Source: CAD feature listing. Evaluate the final solid. Frame: model axes, mm. Coordinates: 2 decimals unless noted, no trailing zeros. Order: outer loops, then holes, each group sorted by start corner. A loop starts at its lowest first (then second) coordinate and runs counter-clockwise, first axis right, second up.
```python
from build123d import *

# Parameters (mm, degrees)
SKETCH1_R               = 6
SKETCH1_R_2             = 15
BOSS_EXTRUDE1_DEPTH     = 5
FILLET1_R               = 5
SKETCH3_R               = 2.1
CUT_EXTRUDE1_DEPTH      = 352.212186577
CIRPATTERN1_COUNT       = 4
CUT_EXTRUDE2_DEPTH      = 352.212186577
CUT_EXTRUDE2_DEPTH_BACK = 352.212186577
SKETCH4_R               = 1.6
SKETCH5_R               = 1.6
SKETCH5_R_2             = 12.5
CUT_EXTRUDE3_DEPTH      = 352.212186577
SKETCH7_R               = 2.2
CUT_EXTRUDE5_DEPTH      = 352.212186577
LPATTERN1_COUNT         = 2
LPATTERN1_PITCH         = 100
CUT_EXTRUDE4_DEPTH      = 352.212186577
CUT_EXTRUDE4_DEPTH_BACK = 352.212186577


with BuildPart() as part:
    # Sketch1 → Boss-Extrude1 (new, symmetric)
    with BuildSketch(Plane(origin=(0, 0, 0), x_dir=(1, 0, 0), z_dir=(0, 1, 0))):
        with BuildLine():
            Line((35, 0), (35, 35))
            Line((35, 35), (300, 35))
            ThreePointArc((300, 35), (335, 70), (300, 105))
            Line((300, 105), (-35, 105))
            Line((-35, 105), (-35, 0))
            ThreePointArc((-35, 0), (0, -35), (35, 0))
        make_face()
        with Locations(Location((0, 0, 0), (0, 0, 270))):
            Circle(SKETCH1_R, mode=Mode.SUBTRACT)
        with Locations(Location((300, 70, 0), (0, 0, 270))):
            Circle(SKETCH1_R_2, mode=Mode.SUBTRACT)
    extrude(amount=BOSS_EXTRUDE1_DEPTH, both=True)

    # Fillet1
    fillet1_edges = [part.edges().sort_by_distance(p)[0] for p in [
        (-35, 0, -105),
        (35, 0, -35),
    ]]
    fillet(fillet1_edges, radius=FILLET1_R)

    # Sketch3 → Cut-Extrude1 (cut, symmetric)
    with BuildSketch(Plane(origin=(0, 5, 0), x_dir=(1, 0, 0), z_dir=(0, 1, 0))):
        with Locations(Location((0, -12, 0), (0, 0, 270))):
            Circle(SKETCH3_R)
    cut_extrude1 = extrude(amount=CUT_EXTRUDE1_DEPTH, both=True, mode=Mode.SUBTRACT)

    # CirPattern1: Cut-Extrude1 ×4 about axis
    cirpattern1_axis = Axis((0, 0, 0), (0, 1, 0))
    for i in range(1, CIRPATTERN1_COUNT):
        add(cut_extrude1.rotate(cirpattern1_axis, i * 360 / CIRPATTERN1_COUNT), mode=Mode.SUBTRACT)

    # Sketch4 → Cut-Extrude2 (cut, two sides: drawn at the far end of the back side and taken through both)
    with BuildSketch(Plane(origin=(0, 5, 0), x_dir=(1, 0, 0), z_dir=(0, 1, 0)).offset(-CUT_EXTRUDE2_DEPTH_BACK)):
        with Locations(Location((230, 95, 0), (0, 0, 270))):
            Circle(SKETCH4_R)
        with Locations(Location((240, 95, 0), (0, 0, 270))):
            Circle(SKETCH4_R)
        with Locations(Location((230, 45, 0), (0, 0, 270))):
            Circle(SKETCH4_R)
        with Locations(Location((240, 45, 0), (0, 0, 270))):
            Circle(SKETCH4_R)
        with Locations(Location((-25, 72.5, 0), (0, 0, 270))):
            Circle(SKETCH4_R)
        with Locations(Location((25, 72.5, 0), (0, 0, 270))):
            Circle(SKETCH4_R)
        with Locations(Location((-25, 62.5, 0), (0, 0, 270))):
            Circle(SKETCH4_R)
        with Locations(Location((25, 62.5, 0), (0, 0, 270))):
            Circle(SKETCH4_R)
        with Locations(Location((130, 95, 0), (0, 0, 270))):
            Circle(SKETCH4_R)
        with Locations(Location((140, 95, 0), (0, 0, 270))):
            Circle(SKETCH4_R)
        with Locations(Location((130, 45, 0), (0, 0, 270))):
            Circle(SKETCH4_R)
        with Locations(Location((140, 45, 0), (0, 0, 270))):
            Circle(SKETCH4_R)
    extrude(amount=CUT_EXTRUDE2_DEPTH + CUT_EXTRUDE2_DEPTH_BACK, mode=Mode.SUBTRACT)

    # Sketch5 → Cut-Extrude3 (cut, symmetric)
    with BuildSketch(Plane(origin=(0, 5, 0), x_dir=(1, 0, 0), z_dir=(0, 1, 0))):
        with Locations(Location((174.5, 85.5, 0), (0, 0, 270))):
            Circle(SKETCH5_R)
        with Locations(Location((174.5, 54.5, 0), (0, 0, 270))):
            Circle(SKETCH5_R)
        with Locations(Location((205.5, 54.5, 0), (0, 0, 270))):
            Circle(SKETCH5_R)
        with Locations(Location((205.5, 85.5, 0), (0, 0, 270))):
            Circle(SKETCH5_R)
        with Locations(Location((190, 70, 0), (0, 0, 270))):
            Circle(SKETCH5_R_2)
        with BuildLine():
            Line((223, 95), (223, 45))
            ThreePointArc((223, 45), (220, 42), (217, 45))
            Line((217, 45), (217, 95))
            ThreePointArc((217, 95), (220, 98), (223, 95))
        make_face()
    cut_extrude3 = extrude(amount=CUT_EXTRUDE3_DEPTH, both=True, mode=Mode.SUBTRACT)

    # Sketch7 → Cut-Extrude5 (cut, through all)
    with BuildSketch(Plane(origin=(0, 5, 0), x_dir=(1, 0, 0), z_dir=(0, 1, 0))):
        with Locations(Location((190, 87.5, 0), (0, 0, 270))):
            Circle(SKETCH7_R)
        with Locations(Location((172.5, 70, 0), (0, 0, 270))):
            Circle(SKETCH7_R)
        with Locations(Location((190, 52.5, 0), (0, 0, 270))):
            Circle(SKETCH7_R)
        with Locations(Location((207.5, 70, 0), (0, 0, 270))):
            Circle(SKETCH7_R)
    cut_extrude5 = extrude(amount=-CUT_EXTRUDE5_DEPTH, mode=Mode.SUBTRACT)

    # LPattern1: Cut-Extrude3, Cut-Extrude5 ×2
    with Locations(*[(-i * LPATTERN1_PITCH, 0, 0) for i in range(1, LPATTERN1_COUNT)]):
        add(cut_extrude3, mode=Mode.SUBTRACT)
        add(cut_extrude5, mode=Mode.SUBTRACT)

    # Sketch6 → Cut-Extrude4 (cut, two sides: drawn at the far end of the back side and taken through both)
    with BuildSketch(Plane(origin=(0, 5, 0), x_dir=(1, 0, 0), z_dir=(0, 1, 0)).offset(-CUT_EXTRUDE4_DEPTH_BACK)):
        with BuildLine():
            Line((-25, 95), (55, 95))
            ThreePointArc((55, 95), (60, 90), (55, 85))
            Line((55, 85), (-25, 85))
            ThreePointArc((-25, 85), (-30, 90), (-25, 95))
        make_face()
    extrude(amount=CUT_EXTRUDE4_DEPTH + CUT_EXTRUDE4_DEPTH_BACK, mode=Mode.SUBTRACT)


solid = part.part
```
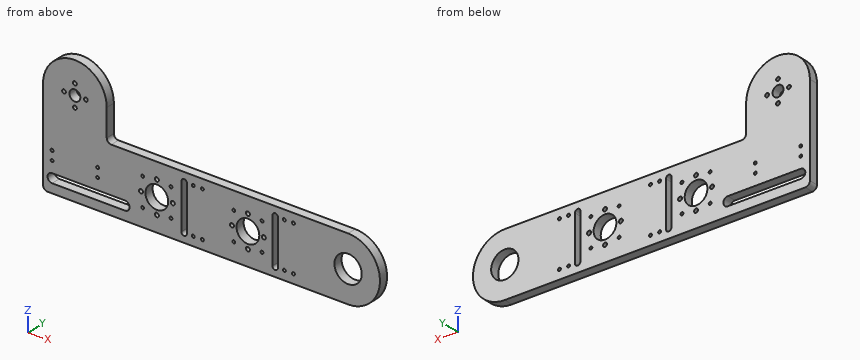
1. Section query C-C, the plane z = -19.5. Output: boundary loops of the cut face in (x, y).
2. Contact query for a flat-ended pin moving along its axis: P1, Ø2, axis at x = 172, y = 0.5, coming from the +Z side. Output: stop coordinate, or through.
3. Material intervals for line 1 along Z through (x, y) = (230, -2.5); line 2 along Z through (x, y) = (25, -0.5); line 3 along X through (y, z) = (-0.75, -75), sorted ascending.
4. Section query B-B, the plane x = 153. Output: boundary loops of the cut face in (y, z).
5. Section query A-A, the plane y = 0.5. Count the separate pieces of the cut face and the enclosed holes in it, plus the area to 3 significant figures.
Answer key:
1. outline: (-35, -5) - (35, -5) - (35, 5) - (-35, 5) - close
2. P1: stops at z = -35
3. line 1: z = -105 to -96.6, -93.4 to -46.6, -43.4 to -35
3. line 2: z = -105 to -95, -85 to -74.1, -70.9 to -64.1, -60.9 to 24.49
3. line 3: x = -35 to 78.54, 101.46 to 117, 123 to 178.54, 201.46 to 217, 223 to 285.86, 314.14 to 334.64
4. outline: (-5, -105) - (5, -105) - (5, -35) - (-5, -35) - close
5. separate pieces: 1
5. enclosed holes: 39
5. area: 26,100 mm2
